from build123d import *

# Parameters (mm, degrees)
SKETCH2_W                       = 20
SKETCH2_H                       = 20
PCB_DEPTH                       = 1.5
SKETCH3_R                       = 1.5
SIDE_MOUNTING_HOLES_FRAME_DEPTH = 1.5
SKETCH4_R                       = 1
SIDE_MOUNTING_HOLES_DEPTH       = 1.5
SKETCH5_R                       = 2.5
SIDE_INLETS_DEPTH               = 1.5
SKETCH6_W                       = 12
SKETCH6_H                       = 5
BOSS_EXTRUDE3_DEPTH             = 8
SKETCH7_W                       = 7
SKETCH7_H                       = 7
BOSS_EXTRUDE4_DEPTH             = 5
SKETCH8_R                       = 1.522673679
CUT_EXTRUDE3_DEPTH              = 0.5
SKETCH9_W                       = 5
SKETCH9_H                       = 3.5
BOSS_EXTRUDE5_DEPTH             = 1


with BuildPart() as part:
    # Sketch2 → pcb (new body)
    with BuildSketch(Plane(origin=(0, 0, 0), x_dir=(1, 0, 0), z_dir=(0, 1, 0))):
        Rectangle(SKETCH2_W, SKETCH2_H)
    extrude(amount=PCB_DEPTH)

    # Sketch3 → side mounting holes frame (add)
    with BuildSketch(Plane(origin=(0, 1.5, 0), x_dir=(1, 0, 0), z_dir=(0, 1, 0))):
        with Locations((-10, 0)):
            Circle(SKETCH3_R)
        with Locations((10, 0)):
            Circle(SKETCH3_R)
    extrude(amount=-SIDE_MOUNTING_HOLES_FRAME_DEPTH)

    # Sketch4 → side mounting holes (cut)
    with BuildSketch(Plane(origin=(0, 1.5, 0), x_dir=(1, 0, 0), z_dir=(0, 1, 0))):
        with Locations((-10, 0)):
            Circle(SKETCH4_R)
        with Locations((10, 0)):
            Circle(SKETCH4_R)
    extrude(amount=-SIDE_MOUNTING_HOLES_DEPTH, mode=Mode.SUBTRACT)

    # Sketch5 → side inlets (cut)
    with BuildSketch(Plane(origin=(0, 1.5, 0), x_dir=(1, 0, 0), z_dir=(0, 1, 0))):
        with Locations((0, 10)):
            Circle(SKETCH5_R)
        with Locations((0, -10)):
            Circle(SKETCH5_R)
    extrude(amount=-SIDE_INLETS_DEPTH, mode=Mode.SUBTRACT)

    # Sketch6 → Boss-Extrude3 (add)
    with BuildSketch(Plane(origin=(0, 1.5, 0), x_dir=(1, 0, 0), z_dir=(0, 1, 0))):
        with Locations((0, -6.5)):
            Rectangle(SKETCH6_W, SKETCH6_H)
    extrude(amount=BOSS_EXTRUDE3_DEPTH)

    # Sketch7 → Boss-Extrude4 (add)
    with BuildSketch(Plane(origin=(0, 1.5, 0), x_dir=(1, 0, 0), z_dir=(0, 1, 0))):
        with Locations((6, 5.738753886)):
            Rectangle(SKETCH7_W, SKETCH7_H)
    extrude(amount=BOSS_EXTRUDE4_DEPTH)

    # Sketch8 → Cut-Extrude3 (cut)
    with BuildSketch(Plane(origin=(0, 6.5, 0), x_dir=(1, 0, 0), z_dir=(0, 1, 0))):
        with Locations((6, 5.738753886)):
            Circle(SKETCH8_R)
    extrude(amount=-CUT_EXTRUDE3_DEPTH, mode=Mode.SUBTRACT)

    # Sketch9 → Boss-Extrude5 (add)
    with BuildSketch(Plane(origin=(0, 1.5, 0), x_dir=(1, 0, 0), z_dir=(0, 1, 0))):
        with Locations((-0.5, -0.582791265)):
            Rectangle(SKETCH9_W, SKETCH9_H)
    extrude(amount=BOSS_EXTRUDE5_DEPTH)


solid = part.part
Here's how the part is built. I have some questions about the finished solid (model axes, mm). A direction names the side the tool comes from. Give positions to 0.01 mm unless a question says otherwise; leave off trailing zeros. Order: outer loops, then holes, each group sorted by start corner. A loop starts at its lowest first (then second) coordinate and runs counter-clockwise, first axis right, second up. Notation, with made-up numbers: M -28.75,41 L 23.25,41 A16 cw 23.25,59 Z; hole C -5.5,51.5 d6. An arc over 180 degrees is marked long. Answer as a JSON object with one key per item and string values. Group by question number.
1) Suppose I cut it at A-A, the plane y = 3.25. Write out the boundary of the cut face in (x, z), plus the area to 3 significant figures.
2) We'd pull the mould along X, two halves only. Please class faces 1 (the flat face through (-1, 2, 2.333)), 2 (the cylindrical face through (-0.1, 0.8, -7.5)), 3 (the flat face through (9.5, 4, -6)): pulls with the +X half, pulls with the -X half, needs draft (parallel to the pull), parting line crosses it, or undercut.
3) Suppose I cut it at B-B, the plane z = 0. Write out the boundary of the cut face in (x, y), plus the area to 3 significant figures.
4) Please list where these lines run through material, in increasing order: L1, parallel to X at y = 0.7, z = 0; L2, parallel to Y at x = -8.5, z = -8; L3, parallel to X at y = 5.75, z = -5.25. Write a range as [from, to].
5) Suppose I cut it at D-D, the plane z = 5.75. Write out the boundary of the cut face in (x, y).
6) On a 3-axis mill with a long thin cutter (end or side, diameter ignored), from which of +Z, -Z, +X, -X, +Y, -Y can I reach the whole of each face in a straight line? I mean faces 4 (the flat face through (0, 5, 4)), 5 (the flat face through (4, 6.5, -6)), 6 (the flat face through (6, 6, -6)). Say none if no direction works.
7) I'm going to push flat-ended pins straight in: pin 1 Ø1.5 at (y, z) = (7.5, 6) entering from -X; pin 2 Ø0.8 at (y, z) = (2, 0) entering from +X; pin 3 Ø3 at (x, z) = (3, -6) entering from +Y. Where does each tip first touch, or does it pass through?
8) Suppose I cut it at C-C, the plane x = 1.5. Write out the boundary of the cut face in (y, z), plus the area to 3 significant figures.
Results found:
{
 "1": {"outline": "M -6,4 L 6,4 L 6,9 L -6,9 Z; M 2.5,-9.24 L 9.5,-9.24 L 9.5,-2.24 L 2.5,-2.24 Z", "area": "109 mm²"},
 "2": {"face 1": "needs draft", "face 2": "undercut", "face 3": "pulls with the +X half"},
 "3": {"outline": "M -11.5,0 L -11,0 L -11,1.5 L -11.5,1.5 Z; M -9,0 L 9,0 L 9,1.5 L 2,1.5 L 2,2.5 L -3,2.5 L -3,1.5 L -9,1.5 Z; M 11,0 L 11.5,0 L 11.5,1.5 L 11,1.5 Z", "area": "33.5 mm²"},
 "4": {"L1": "[-11.5, -11], [-9, 9], [11, 11.5]", "L2": "[0, 1.5]", "L3": "[2.5, 9.5]"},
 "5": {"outline": "M -10,0 L 10,0 L 10,1.5 L 6,1.5 L 6,9.5 L -6,9.5 L -6,1.5 L -10,1.5 Z"},
 "6": {"face 4": "+X, -X, +Y", "face 5": "-Z, +X, -X, +Y", "face 6": "+Y"},
 "7": {"pin 1": "x = -6", "pin 2": "x = 2", "pin 3": "y = 6.5"},
 "8": {"outline": "M 0,-8 L 1.5,-8 L 1.5,-1.17 L 2.5,-1.17 L 2.5,2.33 L 1.5,2.33 L 1.5,4 L 9.5,4 L 9.5,9 L 1.5,9 L 1.5,8 L 0,8 Z", "area": "67.5 mm²"}
}
